Work out the finished part from the listing and answer in its coordinate system (mm). Face numbers are marked on the shaded views. A direction names the side the tool comes from. Give positions to 0.01 mm unless a question says otherwise; leave off trailing zeros. Loops run counter-clockwise (first coordinate to the right, second up) from the corner with the lowest first, then second, coordinate; pieces in that order, holes last. Notation, with made-up numbers: M 1,-35.5 L 48,-35.5 A29 ccw 48,-6.5 Z; hole C -18,56 d4. An arc over 180 degrees is marked long. Use a Markdown table: item, result.
```python
from build123d import *

# Parameters (mm, degrees)
F0_R     = 7.9375
F0_R_2   = 12.7
F0_R_3   = 6.35
F1_DEPTH = 6.35
F2_DEPTH = 31.75


with BuildPart() as f1:
    # F0 (on Front) → F1 (new body, symmetric)
    with BuildSketch(Plane.XZ):
        with BuildLine():
            ThreePointArc((82.55, -7.463384), (50.109619, 24.279109), (19.080024, -8.843819))
            ThreePointArc((19.080024, -8.843819), (17.762053, -12.344458), (14.322027, -13.813384))
            Line((14.322027, -13.813384), (0, -13.813384))
            Line((0, -13.813384), (-14.322027, -13.813384))
            ThreePointArc((-14.322027, -13.813384), (-17.762053, -12.344458), (-19.080024, -8.843819))
            ThreePointArc((-19.080024, -8.843819), (-50.109619, 24.279109), (-82.55, -7.463384))
            Line((-82.55, -7.463384), (-82.55, -34.931994))
            ThreePointArc((-82.55, -34.931994), (-83.623483, -37.944063), (-86.36, -39.598272))
            ThreePointArc((-86.36, -39.598272), (-101.503534, -60.17808), (-82.55, -77.313384))
            Line((-82.55, -77.313384), (-53.975, -77.313384))
            ThreePointArc((-53.975, -77.313384), (-47.239808, -80.103192), (-44.45, -86.838384))
            Line((-44.45, -86.838384), (-44.45, -93.188384))
            ThreePointArc((-44.45, -93.188384), (-41.660192, -99.923576), (-34.925, -102.713384))
            Line((-34.925, -102.713384), (-19.030211, -102.713384))
            Line((-19.030211, -102.713384), (-19.030211, -90.013384))
            ThreePointArc((-19.030211, -90.013384), (-0.516209, -70.970926), (19.039627, -88.941812))
            Line((19.039627, -88.941812), (19.030211, -102.713384))
            Line((19.030211, -102.713384), (34.925, -102.713384))
            ThreePointArc((34.925, -102.713384), (41.660192, -99.923576), (44.45, -93.188384))
            Line((44.45, -93.188384), (44.45, -86.838384))
            ThreePointArc((44.45, -86.838384), (47.239808, -80.103192), (53.975, -77.313384))
            Line((53.975, -77.313384), (82.55, -77.313384))
            ThreePointArc((82.55, -77.313384), (101.503534, -60.17808), (86.36, -39.598272))
            ThreePointArc((86.36, -39.598272), (83.623483, -37.944063), (82.55, -34.931994))
            Line((82.55, -34.931994), (82.55, -7.463384))
        make_face()
        with Locations((-82.55, -58.263384)):
            Circle(F0_R, mode=Mode.SUBTRACT)
        with Locations((0, -42.388384)):
            Circle(F0_R_2, mode=Mode.SUBTRACT)
        with Locations((82.55, -58.263384)):
            Circle(F0_R, mode=Mode.SUBTRACT)
        with Locations((-50.8, -7.463384)):
            Circle(F0_R_2, mode=Mode.SUBTRACT)
        with Locations((50.8, -7.463384)):
            Circle(F0_R_2, mode=Mode.SUBTRACT)
        with Locations((82.55, -58.263384)):
            Circle(F0_R)
        with Locations((82.55, -58.263384)):
            Circle(F0_R_3, mode=Mode.SUBTRACT)
        with Locations((-82.55, -58.263384)):
            Circle(F0_R)
        with Locations((-82.55, -58.263384)):
            Circle(F0_R_3, mode=Mode.SUBTRACT)
    extrude(amount=F1_DEPTH, both=True)

    # F0 (on Front) → F2 (join)
    with BuildSketch(Plane.XZ):
        with Locations((-82.55, -58.263384)):
            Circle(F0_R)
        with Locations((-82.55, -58.263384)):
            Circle(F0_R_3, mode=Mode.SUBTRACT)
        with Locations((82.55, -58.263384)):
            Circle(F0_R)
        with Locations((82.55, -58.263384)):
            Circle(F0_R_3, mode=Mode.SUBTRACT)
    extrude(amount=F2_DEPTH)


solid = f1.part
```
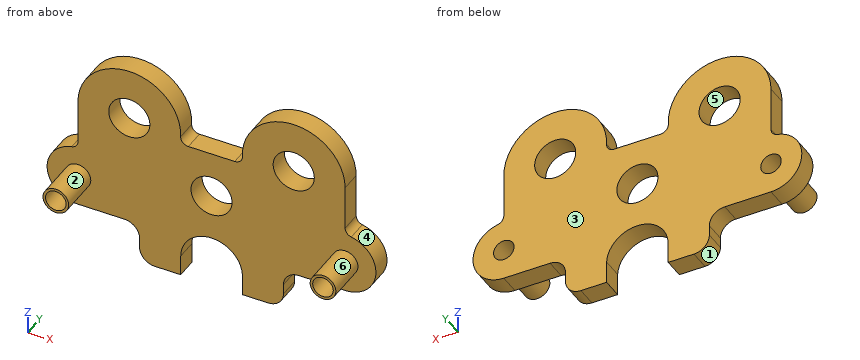
(1) A cutting plane is placed at A-A (x = -50.8). Write down the section's boundary in (y, z).
Entries:
| item | result |
|---|---|
| outline | M -6.35,-77.86 L 6.35,-77.86 L 6.35,-20.16 L -6.35,-20.16 Z; M -6.35,5.24 L 6.35,5.24 L 6.35,24.29 L -6.35,24.29 Z |
(2) A cutting plane is placed at D-D (x = -79). Write down the section's boundary in (y, z), and give its area (3 significant figures).
Entries:
| item | result |
|---|---|
| outline | M -31.75,-65.36 L -6.35,-65.36 L -6.35,-77.31 L 6.35,-77.31 L 6.35,-63.53 L -31.75,-63.53 Z; M -31.75,-53 L 6.35,-53 L 6.35,7.13 L -6.35,7.13 L -6.35,-51.16 L -31.75,-51.16 Z |
| area | 1,030 mm² |
(3) Which of the six approach directions +Z, -Z, +X, -X, +Y, -Y give full straight-line access (tool end or side, diameter ignored) to the marked faces 5 and 6?
Entries:
| item | result |
|---|---|
| face 5 | +Y, -Y |
| face 6 | -Y |
(4) The mould has two halves that part along X. Classify the marked faces 1, 2, 3 and 4: released by +X, released by -X, zero draft, split by the parting line, or undercut.
Entries:
| item | result |
|---|---|
| face 1 | released by -X |
| face 2 | undercut |
| face 3 | zero draft |
| face 4 | released by +X |
(5) A cutting plane is placed at C-C (z = -27.5). Write down the section's boundary in (x, y).
Entries:
| item | result |
|---|---|
| outline | M -82.55,-6.35 L 82.55,-6.35 L 82.55,6.35 L -82.55,6.35 Z |
(6) A cutting plane is placed at B-B (y = -10). Count the separate pieces of the cut face and the enclosed holes in it, and give its area (3 significant figures).
Entries:
| item | result |
|---|---|
| separate pieces | 2 |
| enclosed holes | 2 |
| area | 143 mm² |
(7) Consider probe 1 along X at (y, z) = (2, -16); probe 2 along Y at (x, z) = (-46.5, -36); probe 3 along Z at (x, y) = (5.5, 1.5). Determine where each line is inside the solid, lowest interval first. Write a range as [from, to].
Entries:
| item | result |
|---|---|
| probe 1 | x = [-82.55, -60.2], [-41.4, 41.4], [60.2, 82.55] |
| probe 2 | y = [-6.35, 6.35] |
| probe 3 | z = [-71.77, -53.84], [-30.94, -13.81] |
(8) Given P1, Ø5, axis at y = 0, z = -89, coming from the -X side; P2, Ø6.5, axis at y = -3, z = -98, coming from the +X side; P3, Ø4, axis at y = -2.5, z = -18, coming from the +X side; P4, Ø14.5, axis at x = 82.55, z = -58.26, coming from the -Y side, each flat-ended and moving along its own axis, determine where each tip first touches the part or whether it passes through.
Entries:
| item | result |
|---|---|
| P1 | stops at x = -44.46 |
| P2 | stops at x = 44.32 |
| P3 | stops at x = 82.55 |
| P4 | stops at y = -31.75 |
